The model under review builds one solid part; all positions refer to its coordinate system, in mm. Give positions to 0.01 mm unless a question says otherwise; leave off trailing zeros. Loops run counter-clockwise (first coordinate to the right, second up) from the corner with the lowest first, then second, coordinate; pieces in that order, holes last. Notation, with made-up numbers: (78, -13) -> (113, -13) arc R9 ccw to (113, -8) -> close; hole circle Ø6 at (49.5, 70.25). An arc over 180 degrees is marked (long way). Write each question's results on one line, items separated by ' | '. Start each with the question number.
Q1. Wall thickness on L1, parallel to X at y = 1.5, z = -40; L2, parallel to Z at x = -21.5, y = 8.75; L3, parallel to Z at x = -2, y = 5.75: over which ranges is each line inside the solid? List them lowest first. Write a range as [from, to].
Q2. We need section A-A (y = 6.5). Write out the cut boundary in (x, z), plus the area to 3 significant figures.
Q3. We need section C-C (z = -44). Write out the cut boundary in (x, y).
Q4. We need section D-D (x = -29). Write out the cut boundary in (y, z).
Q5. Insertion check: pin 1 Ø1 at (x, y) = (-23.5, 5) entering from -Z; pin 2 Ø3 at (x, y) = (-24.5, 5) entering from -Z. Each pin has a flat end and moves straight along its axis. Give the tip position at first contact, or say it passes through.
Q6. We need section B-B (x = -6). Write out the cut boundary in (y, z).
Autodesk Inventor part; units mm, degrees
ref_plane "YZ Plane" through (0, 0, 0) normal (1, 0, 0) x (0, 1, 0)
ref_plane "XZ Plane" through (0, 0, 0) normal (0, 1, 0) x (-1, 0, 0)
ref_plane "XY Plane" through (0, 0, 0) normal (0, 0, 1) x (1, 0, 0)
sketch "Sketch1" plane through (0, 0, 0) normal (0, 1, 0) x (-1, 0, 0)
  line L0 (0, 0) -> (38.1, 0)
  line L1 (38.1, 0) -> (38.1, -50.8)
  line L2 (38.1, -50.8) -> (0, -50.8)
  line L3 (0, -50.8) -> (0, 0)
  dimension "d0" = 38.1
  dimension "d1" = 50.8
extrude "Extrusion1" add sketch "Sketch1" along normal blind 10.16
fillet "Fillet1" radius 12.7 3 edges at (0, 5.08, -50.8) (-38.1, 5.08, -50.8) (-19.05, 10.16, -50.8)
properties part number "EndStopMounts"
Output:
1) L1: [-37.96, -0.14] | L2: [-44.17, 0] | L3: [-44.94, 0]
2) outline: (-38.1, -38.1) arc R12.7 ccw to (-34.18, -47.28) -> (-3.92, -47.28) arc R12.7 ccw to (0, -38.1) -> (0, 0) -> (-38.1, 0) -> close | area: 1,780 mm2
3) outline: (-36.65, 0) -> (-1.45, 0) -> (-1.45, 8.84) -> (-36.65, 8.84) -> close
4) outline: (0, -50.28) -> (1.84, -50.28) arc R12.7 ccw to (10.16, -38.36) -> (10.16, 0) -> (0, 0) -> close
5) pin 1: z = -48.93 | pin 2: z = -49.53
6) outline: (0, -48.89) -> (4.56, -48.89) arc R12.7 ccw to (10.16, -38.36) -> (10.16, 0) -> (0, 0) -> close
